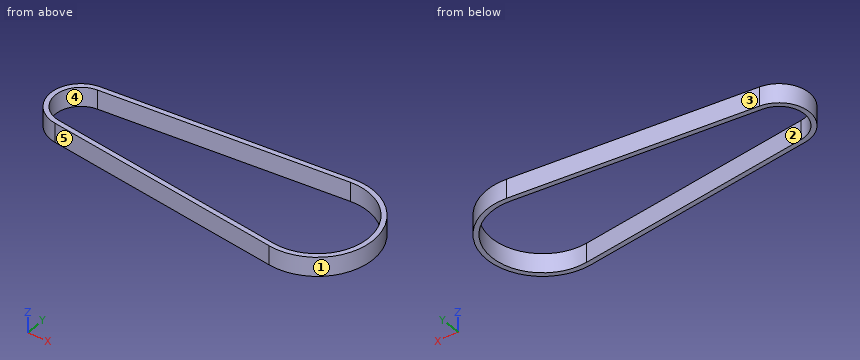
Autodesk Inventor part; units mm, degrees
ref_plane "YZ Plane" through (0, 0, 0) normal (1, 0, 0) x (0, 1, 0)
ref_plane "XZ Plane" through (0, 0, 0) normal (0, 1, 0) x (-1, 0, 0)
ref_plane "XY Plane" through (0, 0, 0) normal (0, 0, 1) x (1, 0, 0)
sketch "Sketch3" plane through (0, 0, 0) normal (0, 1, 0) x (-1, 0, 0)
  line L0 (0, 0) -> (8, 0) construction
  line L1 (8, 0) -> (8, -3)
  line L2 (8, -3) -> (9.5, -3)
  line L3 (9.5, -3) -> (9.5, 3)
  line L4 (9.5, 3) -> (8, 3)
  line L5 (8, 3) -> (8, 0)
  dimension "d9" = 1.5
  dimension "d10" = 6
  dimension "d11" = 8
sketch "Sketch1" plane through (0, 0, 0) normal (0, 0, 1) x (1, 0, 0)
  line L0 (0, 0) -> (74.5, 0) construction
  arc A0 (72.7819, -15.9075) -> (72.7819, 15.9075) centre (74.5, 0) ccw
  arc A1 (-0.8591, 7.9537) -> (-0.8591, -7.9537) centre (0, 0) ccw
  line L1 (-0.8591, 7.9537) -> (72.7819, 15.9075)
  line L2 (-0.8591, -7.9537) -> (72.7819, -15.9075)
  dimension "d0" = 74.5
  dimension "d2" = 16
  dimension "d8" = 32
sweep "Sweep1" add profiles "Sketch3" path "Sketch1"
properties part number "Conrod"
Source: CAD feature listing. Evaluate the final solid. Frame: model axes, mm. Face numbers are marked on the shaded views. A direction names the side the tool comes from. Give positions to 0.01 mm unless a question says otherwise; leave off trailing zeros. Order: outer loops, then holes, each group sorted by start corner. A loop starts at its lowest first (then second) coordinate and runs counter-clockwise, first axis right, second up. Notation, with made-up numbers: (67, 61.25) -> (113, 61.25) arc R28 ccw to (113, 82.25) -> close; hole circle Ø10 at (-18, -39). An arc over 180 degrees is marked (long way). Use a Markdown table: item, result.
1) Reachability of the marked faces 4 and 5 from +Z, -Z, +X, -X, +Y, -Y: full face, straight path, thin tool, end or side. Return the list, or none.
Answer list:
| item | result |
|---|---|
| face 4 | +Z, -Z |
| face 5 | +Z, -Z, -X, -Y |
2) Contact query for flat-ended pins moving along their axis: P1, Ø2, axis at y = 4, z = -0.5, coming from the -X side; P2, Ø1.5, axis at y = -8.5, z = 1.5, coming from the +X side. Output: stop coordinate, or through.
Answer list:
| item | result |
|---|---|
| P1 | x = -9.01 |
| P2 | x = 90.19 |
3) Mould query, pull axis Y, two halves, no side actions, for the marked faces 1, 2 and 3. Classes: +Y half, -Y half, draft (parallel to the pull), parting line (faces both ways), or undercut.
Answer list:
| item | result |
|---|---|
| face 1 | parting line |
| face 2 | undercut |
| face 3 | +Y half |
4) Section query A-A, the plane y = 0. Return the cut outline in (x, z).
Answer list:
| item | result |
|---|---|
| outline | (-9.5, -3) -> (-8, -3) -> (-8, 3) -> (-9.5, 3) -> close; (90.5, -3) -> (92, -3) -> (92, 3) -> (90.5, 3) -> close |
5) Section query B-B, the plane x = 74.5. Return the cut outline in (y, z), then the cut area to 3 significant figures.
Answer list:
| item | result |
|---|---|
| outline | (-17.5, -3) -> (-16, -3) -> (-16, 3) -> (-17.5, 3) -> close; (16, -3) -> (17.5, -3) -> (17.5, 3) -> (16, 3) -> close |
| area | 18.0 mm² |
6) Ray query, line 1 along Y through (x, z) = (74.5, -1.4); line 2 along Y through (x, z) = (-2, -2.3); line 3 along X through (y, z) = (4.5, 1.8). Return the intervals inside material, ascending. Write a range as [from, to].
Answer list:
| item | result |
|---|---|
| line 1 | [-17.5, -16], [16, 17.5] |
| line 2 | [-9.29, -7.75], [7.75, 9.29] |
| line 3 | [-8.37, -6.61], [89.85, 91.41] |
7) Section query C-C, the plane z = -0.65. Return the cut outline in (x, y).
Answer list:
| item | result |
|---|---|
| outline | (-1.02, -9.45) -> (72.62, -17.4) arc R17.5 ccw (long way) to (72.62, 17.4) -> (-1.02, 9.45) arc R9.5 ccw to start; hole (-0.86, -7.95) -> (72.78, -15.91) arc R16 ccw (long way) to (72.78, 15.91) -> (-0.86, 7.95) arc R8 ccw to start |
